```python
from build123d import *

# Parameters (mm, degrees)
SKETCH1_R           = 4
BOSS_EXTRUDE2_DEPTH = 10


with BuildPart() as part:
    # Sketch1 → Boss-Extrude2 (new body)
    with BuildSketch(Plane.XY):
        Polygon((-115, 35), (115, 35), (115, 25), (25, 25), (25, 15), (115, 15), (115, -35), (-115, -35), (-115, -25), (-25, -25), (-25, -15), (-115, -15), align=None)
        Circle(SKETCH1_R, mode=Mode.SUBTRACT)
    extrude(amount=BOSS_EXTRUDE2_DEPTH)


solid = part.part
```
The listing builds one solid part. Answer for the finished solid, in the listing's coordinates (mm). A direction names the side the tool comes from. Give positions to 0.01 mm unless a question says otherwise; leave off trailing zeros. Order: outer loops, then holes, each group sorted by start corner. A loop starts at its lowest first (then second) coordinate and runs counter-clockwise, first axis right, second up. Notation, with made-up numbers: (71, 38) - (79, 38) arc R13 cw to (79, 62) - close; hole circle Ø1 at (-37.5, 40). An arc over 180 degrees is marked (long way). Answer in a Markdown table with one row per item. Add a question column.
Q1. The part is cut by section B-B (y = 0). Determine the outline of the cut face in (x, z), then the cut area to 3 significant figures.
Q2. For a pull along X with two mould halves and no side action, classify faces 1 (the flat face through (2, -7, 10)), 2 (the cylindrical face through (-0.867, -3.905, 4.93)), 3 (the flat face through (115, -10, 5)), 4 (the flat face through (-115, 10, 5)) as released by +X, released by -X, zero draft, split by the parting line, or undercut.
Q3. Given P1, Ø5, axis at y = -19.5, z = 3.5, coming from the -X side, flat-ended and moving along its own axis, determine where the tip first touches the part or whether it passes through.
Q4. Which of the six approach directions +Z, -Z, +X, -X, +Y, -Y give full straight-line access (tool end or side, diameter ignored) to faces 5 (the flat face through (71, 25, 5)), 6 (the flat face through (2, -35, 5)), 7 (the flat face through (-25, -20, 5))?
Q5. Find the intervals of material crossed by line 1 along Y through (x, z) = (-96.5, 0.5); line 2 along Y through (x, z) = (0, 5.25); line 3 along X through (y, z) = (17.5, 5), in increasing order. Write a range as [from, to].
Q6. The part is cut by section A-A (x = 0). Determine the outline of the cut face in (y, z).
Q7. The part is cut by section C-C (z = 5.25). Determine the outline of the cut face in (x, y), then the cut area to 3 significant figures.
Determined:
| question | item | result |
|---|---|---|
| 1 | outline | (-115, 0) - (-4, 0) - (-4, 10) - (-115, 10) - close; (4, 0) - (115, 0) - (115, 10) - (4, 10) - close |
| 1 | area | 2,220 mm² |
| 2 | face 1 | zero draft |
| 2 | face 2 | undercut |
| 2 | face 3 | released by +X |
| 2 | face 4 | released by -X |
| 3 | P1 | stops at x = -25 |
| 4 | face 5 | +Z, -Z, +X |
| 4 | face 6 | +Z, -Z, +X, -X, -Y |
| 4 | face 7 | +Z, -Z, -X |
| 5 | line 1 | y = [-35, -25], [-15, 35] |
| 5 | line 2 | y = [-35, -4], [4, 35] |
| 5 | line 3 | x = [-115, 25] |
| 6 | outline | (-35, 0) - (-4, 0) - (-4, 10) - (-35, 10) - close; (4, 0) - (35, 0) - (35, 10) - (4, 10) - close |
| 7 | outline | (-115, -35) - (115, -35) - (115, 15) - (25, 15) - (25, 25) - (115, 25) - (115, 35) - (-115, 35) - (-115, -15) - (-25, -15) - (-25, -25) - (-115, -25) - close; hole circle Ø8 at (0, 0) |
| 7 | area | 14,200 mm² |
